Drawing for the job (mm, zero at the part's lowest x, y, z). Coordinates: 2 decimals unless noted, no trailing zeros. Loops run counter-clockwise (first coordinate to the right, second up) from the corner with the lowest first, then second, coordinate; pieces in that order, holes last. Notation, with made-up numbers: (16.25, 24.25) - (48.25, 24.25) arc R17 ccw to (48.25, 38.25) - close; hole circle Ø8 at (-9, 22.5). An arc over 180 degrees is marked (long way). One line per item, written item: value.
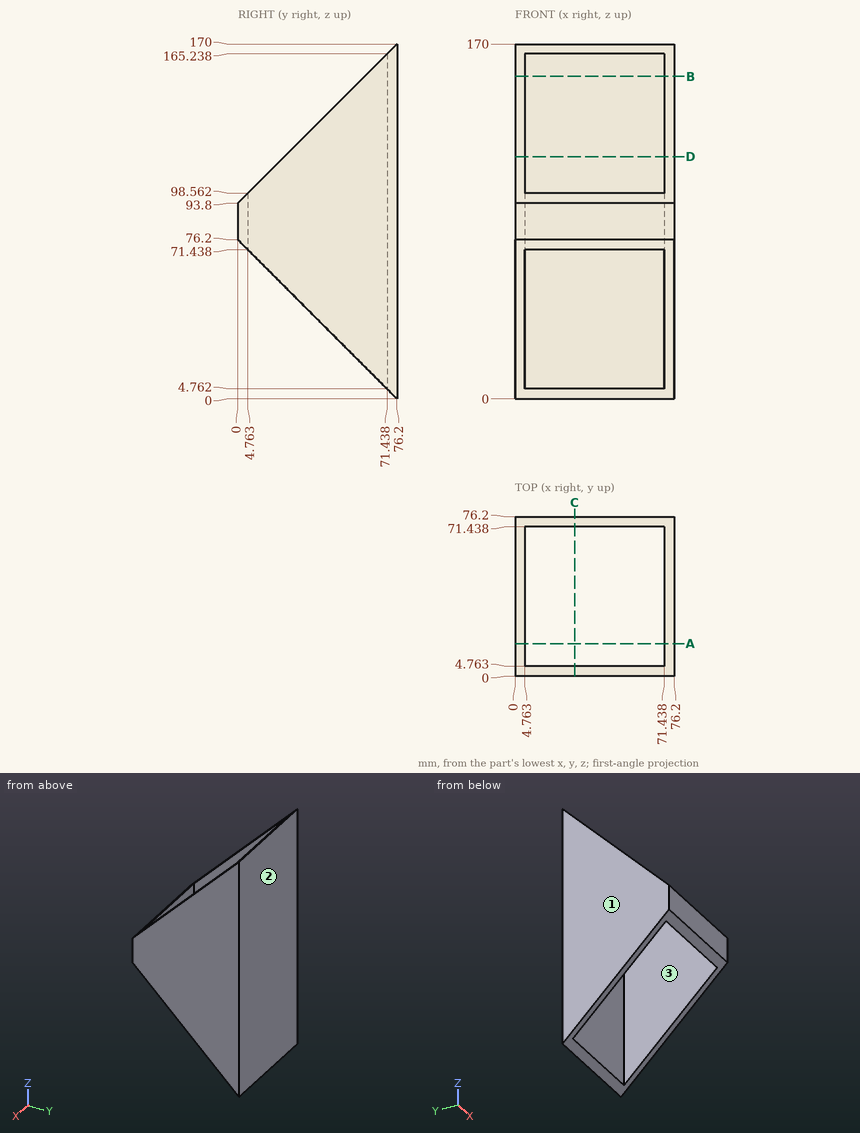
Item 1: Cut at A-A, the plane y = 15.5. Write the cut outline in (x, z).
Check result:
outline: (0, 60.7) - (4.76, 60.7) - (4.76, 109.3) - (0, 109.3) - close; (71.44, 60.7) - (76.2, 60.7) - (76.2, 109.3) - (71.44, 109.3) - close
Item 2: Drop flat-ended pins along their axis: P1, Ø1.5, axis at x = 23.5, z = 97.5, coming from the -Y side; P2, Ø12, axis at x = 13.5, y = 32, coming from the +Z side; P3, Ø3, axis at x = 63, z = 119, coming from the -Y side. Give the stop position or say it passes through.
Check result:
P1: stops at y = 2.95
P2: passes through
P3: stops at y = 71.44
Item 3: Cut at B-B, the plane z = 154.5. Write the cut outline in (x, y), then the cut area to 3 significant figures.
Check result:
outline: (0, 60.7) - (4.76, 60.7) - (4.76, 71.44) - (71.44, 71.44) - (71.44, 60.7) - (76.2, 60.7) - (76.2, 76.2) - (0, 76.2) - close
area: 465 mm^2
Item 4: Cut at C-C, the plane x = 28.5. Write the cut outline in (y, z).
Check result:
outline: (0, 76.2) - (4.76, 71.44) - (4.76, 98.56) - (0, 93.8) - close; (71.44, 4.76) - (76.2, 0) - (76.2, 170) - (71.44, 165.24) - close
Item 5: Pull direction X, two halves, no side cores. Call the marked faces 1, 2 and 3: released by +X, released by -X, zero draft, split by the parting line, or undercut.
Check result:
face 1: released by -X
face 2: zero draft
face 3: undercut
Item 6: Probe probe 1 along Y at (x, z) = (36.5, 89.5); probe 2 along Y at (x, z) = (31, 101). List the from-to ranges inside material, lowest first. Write a range as from..to.
Check result:
probe 1: y = 0..4.76, 71.44..76.2
probe 2: y = 71.44..76.2
Item 7: Cut at D-D, the plane z = 116. Write the cut outline in (x, y), then the cut area to 3 significant figures.
Check result:
outline: (0, 22.2) - (4.76, 22.2) - (4.76, 71.44) - (71.44, 71.44) - (71.44, 22.2) - (76.2, 22.2) - (76.2, 76.2) - (0, 76.2) - close
area: 832 mm^2
